Part model, mm, in its own coordinate system. Face numbers are marked on the shaded views. A direction names the side the tool comes from. Give positions to 0.01 mm unless a question says otherwise; leave off trailing zeros. Order: outer loops, then holes, each group sorted by start corner. A loop starts at its lowest first (then second) coordinate and runs counter-clockwise, first axis right, second up. Notation, with made-up numbers: (2, 26.5) -> (35, 26.5) arc R15 ccw to (35, 32.5) -> close; hole circle Ø5 at (67.25, 3.25). An arc over 180 degrees is marked (long way). Write item = value, one per line. Start each with the question number.
Item 1: Drill centre lines: line 1 along X through (y, z) = (-11.5, 6.5); line 2 along Y through (x, z) = (29, 3.75); line 3 along X through (y, z) = (-17.5, 7.25). Where is each one in solid material? Low to high.
Item 2: Band-saw the part on D-D on y = 3.5. Write the cut outline in (x, z), plus the area to 3 significant figures.
Item 3: Band-saw the part on C-C on y = -16. Write the cut outline in (x, z), plus the area to 3 significant figures.
Item 4: Pull direction Y, two halves, no side cores. Call the marked faces 1, 2 and 3: +Y half, -Y half, draft (parallel to the pull), parting line (faces both ways), or undercut.
Item 5: Tool access for the marked faces 4 and 5: list every direction of +Z, -Z, +X, -X, +Y, -Y with a clear straight run to the whole face (end or side of a thin tool).
Item 6: Band-saw the part on A-A on x = 32.5. Write the cut outline in (y, z), plus the area to 3 significant figures.
Item 7: Flat gauge pins, fed straight in: P1, Ø4, axis at y = 13.5, z = 6.5, coming from the +X side; P2, Ø2, axis at y = 1.5, z = 6, coming from the +X side; P3, Ø3, axis at x = -7.5, z = 7, coming from the +Y side. Where does each tip first touch, or does it go through?
Item 8: Band-saw the part on B-B on z = 4.75. Write the cut outline in (x, y), plus the area to 3 significant figures.
```python
from build123d import *

# Parameters (mm, degrees)
F1_DEPTH = 7.62


# Not quite as in the source:
# - a feature names something its author has since deleted; it is built from what else it names


with BuildPart() as f1:
    # F0 (on Top) → F1 (new body)
    with BuildSketch(Plane.XY):
        with BuildLine():
            ThreePointArc((-12.5356913124, 29.4331641691), (-7.0772530666, 24.60295999), (0, 22.86))
            ThreePointArc((0, 22.86), (7.0772530666, 24.60295999), (12.5356913124, 29.4331641691))
            ThreePointArc((12.5356913124, 29.4331641691), (14.5482221526, 33.5605251185), (15.24, 38.1))
            ThreePointArc((15.24, 38.1), (-4.5394748815, 52.6482221526), (-12.5356913124, 29.4331641691))
        make_face()
        Polygon((5.0038, 29.4331641691), (0, 29.4331641691), (-5.0038, 29.4331641691), (-10.0076, 38.1), (-5.0038, 46.7668358309), (5.0038, 46.7668358309), (10.0076, 38.1), align=None, mode=Mode.SUBTRACT)
        with BuildLine():
            ThreePointArc((27.9917678842, -4.654876327), (23.2845420207, -7.3046359495), (19.7973407305, -11.43))
            ThreePointArc((19.7973407305, -11.43), (17.7681618263, -19.6694390603), (20.4598765718, -27.7168358309))
            ThreePointArc((20.4598765718, -27.7168358309), (37.5350427657, -33.5982221526), (48.2355678842, -19.05))
            ThreePointArc((48.2355678842, -19.05), (41.8273199187, -6.6299454107), (27.9917678842, -4.654876327))
        make_face()
        Polygon((22.9879678842, -19.05), (25.4898678842, -14.7165820845), (27.9917678842, -10.3831641691), (37.9993678842, -10.3831641691), (43.0031678842, -19.05), (37.9993678842, -27.7168358309), (27.9917678842, -27.7168358309), align=None, mode=Mode.SUBTRACT)
        with BuildLine():
            ThreePointArc((-17.7555678842, -19.05), (-18.2748582915, -15.1055977526), (-19.7973407305, -11.43))
            ThreePointArc((-19.7973407305, -11.43), (-23.2845420207, -7.3046359495), (-27.9917678842, -4.654876327))
            ThreePointArc((-27.9917678842, -4.654876327), (-47.4825252222, -23.7813493938), (-20.4598765718, -27.7168358309))
            ThreePointArc((-20.4598765718, -27.7168358309), (-18.4473457316, -23.5894748815), (-17.7555678842, -19.05))
        make_face()
        Polygon((-27.9917678842, -10.3831641691), (-25.4898678842, -14.7165820845), (-22.9879678842, -19.05), (-27.9917678842, -27.7168358309), (-37.9993678842, -27.7168358309), (-43.0031678842, -19.05), (-37.9993678842, -10.3831641691), align=None, mode=Mode.SUBTRACT)
        with BuildLine():
            ThreePointArc((-9.5247205959, -5.4991), (-9.5247205959, 5.4991), (0, 10.9982))
            Line((0, 10.9982), (0, 22.86))
            ThreePointArc((0, 22.86), (-7.0772530666, 24.60295999), (-12.5356913124, 29.4331641691))
            ThreePointArc((-12.5356913124, 29.4331641691), (-17.2521616486, 11.0236496258), (-27.9917678842, -4.654876327))
            ThreePointArc((-27.9917678842, -4.654876327), (-23.2845420207, -7.3046359495), (-19.7973407305, -11.43))
            Line((-19.7973407305, -11.43), (-9.5247205959, -5.4991))
        make_face()
        with BuildLine():
            Line((0, 22.86), (0, 10.9982))
            ThreePointArc((0, 10.9982), (7.7769018008, 7.7769018008), (10.9982, 0))
            ThreePointArc((10.9982, 0), (10.6234454227, -2.8465436218), (9.5247205959, -5.4991))
            Line((9.5247205959, -5.4991), (19.7973407305, -11.43))
            ThreePointArc((19.7973407305, -11.43), (23.2845420207, -7.3046359495), (27.9917678842, -4.654876327))
            ThreePointArc((27.9917678842, -4.654876327), (17.2521616486, 11.0236496258), (12.5356913124, 29.4331641691))
            ThreePointArc((12.5356913124, 29.4331641691), (7.0772530666, 24.60295999), (0, 22.86))
        make_face()
        with BuildLine():
            ThreePointArc((9.5247205959, -5.4991), (0, -10.9982), (-9.5247205959, -5.4991))
            Line((-9.5247205959, -5.4991), (-19.7973407305, -11.43))
            ThreePointArc((-19.7973407305, -11.43), (-18.2748582915, -15.1055977526), (-17.7555678842, -19.05))
            ThreePointArc((-17.7555678842, -19.05), (-18.4473457316, -23.5894748815), (-20.4598765718, -27.7168358309))
            ThreePointArc((-20.4598765718, -27.7168358309), (0, -23.7392913379), (20.4598765718, -27.7168358309))
            ThreePointArc((20.4598765718, -27.7168358309), (17.7681618263, -19.6694390603), (19.7973407305, -11.43))
            Line((19.7973407305, -11.43), (9.5247205959, -5.4991))
        make_face()
    extrude(amount=F1_DEPTH)


solid = f1.part
```
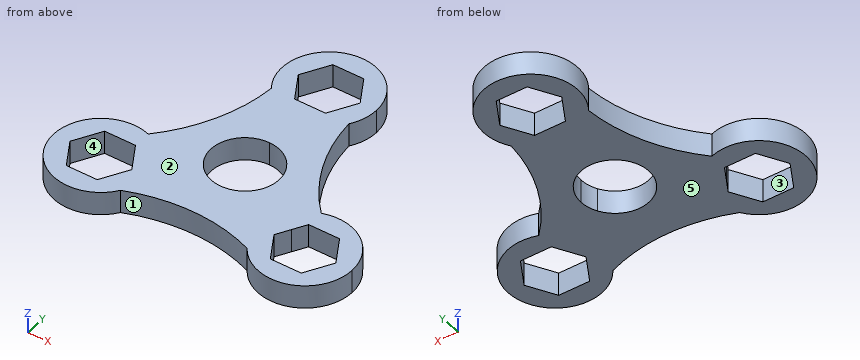
Values found:
q1.line_1 = -46.23 to -38.64, -27.35 to 27.35, 38.64 to 46.23
q1.line_2 = -33.76 to -27.72, -10.38 to -4.34
q1.line_3 = -48.16 to -42.11, -23.88 to 23.88, 42.11 to 48.16
q2.outline = (-21.41, 0) -> (-10.43, 0) -> (-10.43, 7.62) -> (-21.41, 7.62) -> close; (10.43, 0) -> (21.41, 0) -> (21.41, 7.62) -> (10.43, 7.62) -> close
q2.area = 167 mm^2
q3.outline = (-47.93, 0) -> (-41.24, 0) -> (-41.24, 7.62) -> (-47.93, 7.62) -> close; (-24.75, 0) -> (24.75, 0) -> (24.75, 7.62) -> (-24.75, 7.62) -> close; (41.24, 0) -> (47.93, 0) -> (47.93, 7.62) -> (41.24, 7.62) -> close
q3.area = 479 mm^2
q4.face_1 = -Y half
q4.face_2 = draft
q4.face_3 = undercut
q5.face_4 = +Z, -Z
q5.face_5 = -Z, +X, -X, +Y, -Y
q6.outline = (-34.28, 0) -> (-27.72, 0) -> (-27.72, 7.62) -> (-34.28, 7.62) -> close; (-10.38, 0) -> (-3.82, 0) -> (-3.82, 7.62) -> (-10.38, 7.62) -> close
q6.area = 100 mm^2
q7.P1 = 17.04
q7.P2 = 23.53
q7.P3 = 52.11
q8.outline = (-27.99, -4.65) arc R15.24 ccw (long way) to (-20.46, -27.72) arc R54.61 cw to (20.46, -27.72) arc R15.24 ccw (long way) to (27.99, -4.65) arc R54.61 cw to (12.54, 29.43) arc R15.24 ccw (long way) to (-12.54, 29.43) arc R54.61 cw to start; hole (-43, -19.05) -> (-38, -27.72) -> (-27.99, -27.72) -> (-22.99, -19.05) -> (-27.99, -10.38) -> (-38, -10.38) -> close; hole circle Ø22 at (0, 0); hole (-10.01, 38.1) -> (-5, 29.43) -> (5, 29.43) -> (10.01, 38.1) -> (5, 46.77) -> (-5, 46.77) -> close; hole (22.99, -19.05) -> (27.99, -27.72) -> (38, -27.72) -> (43, -19.05) -> (38, -10.38) -> (27.99, -10.38) -> close
q8.area = 2,930 mm^2
